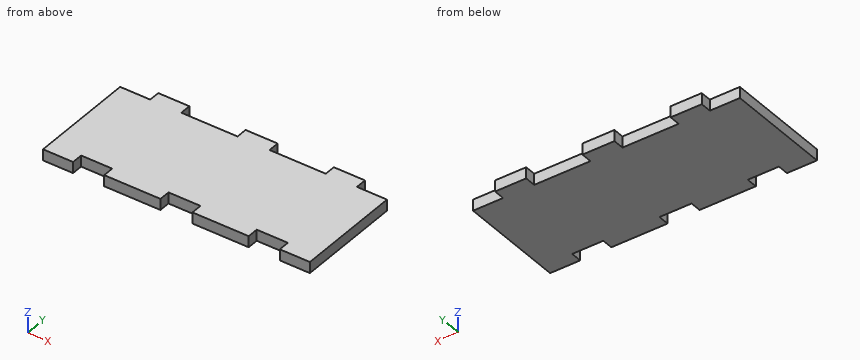
from build123d import *

# Parameters (mm, degrees)
F0_W     = 8.89
F0_H     = 3.175
F0_W_2   = 9.144
F1_DEPTH = 3.175


with BuildPart() as f1:
    # F0 (on Top) → F1 (new body)
    with BuildSketch(Plane.XY):
        with Locations((-25.0698, 16.8275)):
            Rectangle(F0_W, F0_H)
        Polygon((-29.5148, 15.24), (-38.1, 15.24), (-38.1, -15.24), (-29.5148, -15.24), (-29.5148, -12.065), (-20.6248, -12.065), (-20.6248, -15.24), (-4.572, -15.24), (-4.572, -12.065), (4.572, -12.065), (4.572, -15.24), (20.6248, -15.24), (20.6248, -12.065), (29.5148, -12.065), (29.5148, -15.24), (38.1, -15.24), (38.1, 15.24), (29.5148, 15.24), (20.6248, 15.24), (4.572, 15.24), (-4.572, 15.24), (-20.6248, 15.24), align=None)
        with Locations((0, 16.8275)):
            Rectangle(F0_W_2, F0_H)
        with Locations((25.0698, 16.8275)):
            Rectangle(F0_W, F0_H)
    extrude(amount=F1_DEPTH)


solid = f1.part
Can you work these out from the model? Positions are in its coordinate system, mm. Give positions to 0.01 mm unless a question says otherwise; leave off trailing zeros. Order: outer loops, then holes, each group sorted by start corner. A loop starts at its lowest first (then second) coordinate and runs counter-clockwise, first axis right, second up. Notation, with made-up numbers: M 85,83 L 102,83 A12 ccw 102,90 Z; hole C -24,42 d3. An arc over 180 degrees is marked long. One line per item, written item: value.
Item 1: If we section it at A-A on z = 1.65: Write out the boundary of the cut face in (x, y) (3 decimals).
Verdict:
outline: M -38.1,-15.24 L -29.515,-15.24 L -29.515,-12.065 L -20.625,-12.065 L -20.625,-15.24 L -4.572,-15.24 L -4.572,-12.065 L 4.572,-12.065 L 4.572,-15.24 L 20.625,-15.24 L 20.625,-12.065 L 29.515,-12.065 L 29.515,-15.24 L 38.1,-15.24 L 38.1,15.24 L 29.515,15.24 L 29.515,18.415 L 20.625,18.415 L 20.625,15.24 L 4.572,15.24 L 4.572,18.415 L -4.572,18.415 L -4.572,15.24 L -20.625,15.24 L -20.625,18.415 L -29.515,18.415 L -29.515,15.24 L -38.1,15.24 Z
Item 2: Please list where these lines run through material, in increasing order: line 1 (Y direction, x = 16, z = 1.8); line 2 (Y direction, x = -2, z = 1.75) (3 decimals).
Verdict:
line 1: -15.24 to 15.24
line 2: -12.065 to 18.415
Item 3: If we section it at B-B on x = -15: Write out the boundary of the cut face in (y, z) (3 decimals).
Verdict:
outline: M -15.24,0 L 15.24,0 L 15.24,3.175 L -15.24,3.175 Z
Item 4: For pin 1 (1.6 mm diameter, centred on x = -35.5, z = 1.5, fed in from +Y); pin 2 (1 mm diameter, centred on x = 24.5, z = 2, fed in from -Y) (3 decimals); pin 3 (1 mm diameter, centred on y = 16, z = 1.5, fed in from -X), each with a flat end and sliding along its axis, tell me the tip position at first contact or that it passes through.
Verdict:
pin 1: y = 15.24
pin 2: y = -12.065
pin 3: x = -29.51
